Source: CAD feature listing. Evaluate the final solid. Frame: model axes, mm. Face numbers are marked on the shaded views. A direction names the side the tool comes from. Coordinates: 2 decimals unless noted, no trailing zeros. Order: outer loops, then holes, each group sorted by start corner. A loop starts at its lowest first (then second) coordinate and runs counter-clockwise, first axis right, second up. Notation, with made-up numbers: (34, -9) -> (39, -9) arc R33 cw to (39, 29) -> close; hole circle Ø8 at (8.25, 75.25). An arc over 180 degrees is marked (long way). Put each result on its own line as item: value.
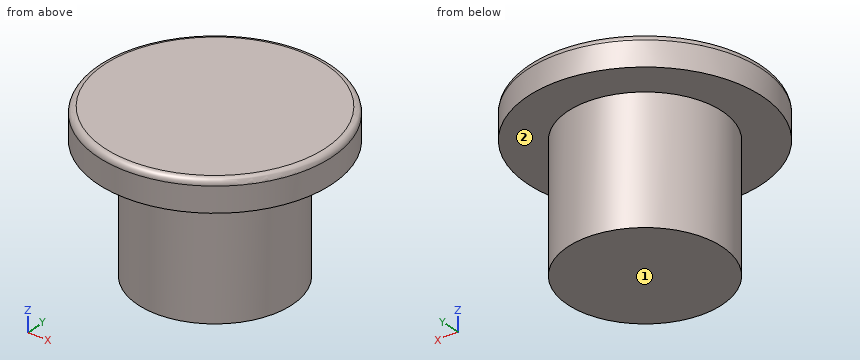
from build123d import *

# Parameters (mm, degrees)
SKETCH1_R           = 7.5
BOSS_EXTRUDE1_DEPTH = 2
SKETCH2_R           = 4.945
BOSS_EXTRUDE2_DEPTH = 10
FILLET2_R           = 0.4


with BuildPart() as part:
    # Sketch1 → Boss-Extrude1 (new body)
    with BuildSketch(Plane.XY):
        Circle(SKETCH1_R)
    extrude(amount=-BOSS_EXTRUDE1_DEPTH)

    # Sketch2 → Boss-Extrude2 (add)
    with BuildSketch(Plane.XY):
        Circle(SKETCH2_R)
    extrude(amount=-BOSS_EXTRUDE2_DEPTH)

    # Fillet2
    fillet2_edges = [part.edges().sort_by_distance(p)[0] for p in [
        (-7.5, 0, 0),
    ]]
    fillet(fillet2_edges, radius=FILLET2_R)


solid = part.part
1. First-contact query: pin 1 (6 mm diameter, centred on y = 4, z = -6, fed in from -X); pin 2 (1.5 mm diameter, centred on x = -4.5, z = -3.5, fed in from +Y); pin 3 (3 mm diameter, centred on x = -0.5, y = 4.5, fed in from +Z); pin 4 (1 mm diameter, centred on x = -0.5, z = -5.5, fed in from -Y) (3 decimals). Flat tips, straight axial feed; report the tip coordinate or a pass-through.
Numbers:
pin 1: stops at x = -4.84
pin 2: stops at y = 3.22
pin 3: stops at z = 0
pin 4: stops at y = -4.945
2. Cut plane A-A on x = 0. Output: boundary loops of the cut face in (y, z) (3 decimals), plus the area to 3 significant figures.
Numbers:
outline: (-7.5, -2) -> (-4.945, -2) -> (-4.945, -10) -> (4.945, -10) -> (4.945, -2) -> (7.5, -2) -> (7.5, -0.4) arc R0.4 ccw to (7.1, 0) -> (-7.1, 0) arc R0.4 ccw to (-7.5, -0.4) -> close
area: 109 mm2
3. Ray query, line 1 along X through (y, z) = (-0.25, -1.5); line 2 along Z through (x, y) = (0.75, 5.25); line 3 along Y through (x, z) = (0, -3.5) (3 decimals). Return the intervals inside material, ascending.
Numbers:
line 1: x = -7.5 to 7.5
line 2: z = -2 to 0
line 3: y = -4.945 to 4.945
4. Cut plane C-C on z = -5.75. Output: boundary loops of the cut face in (x, y) (3 decimals).
Numbers:
outline: circle Ø9.89 at (0, 0)
5. Set-up query: the marked faces 1 and 2. Return all of +Z, -Z, +X, -X, +Y, -Y with unobstructed straight access to the full face (end or side cutting, diameter ignored); none if empty.
Numbers:
face 1: -Z, +X, -X, +Y, -Y
face 2: -Z
